Geometry: final body of the model. Coordinates: model frame, mm. Face numbers are marked on the shaded views. Give positions to 0.01 mm unless a question says otherwise; leave off trailing zeros. Loops run counter-clockwise (first coordinate to the right, second up) from the corner with the lowest first, then second, coordinate; pieces in that order, holes last. Notation, with made-up numbers: M -23,66 L 15,66 A32 cw 15,96 Z; hole C 67.25,50.25 d9. An arc over 180 degrees is marked long. Put each result on its own line as item: value.
```python
from build123d import *

# Parameters (mm, degrees)
F0_W     = 50.8
F0_H     = 101.6
F0_R     = 7.62
F1_DEPTH = 12.7
F2_R     = 5.08
F3_R     = 5.313605
F4_DEPTH = 25.4


with BuildPart() as f1:
    # F0 (on Front) → F1 (new body, symmetric)
    with BuildSketch(Plane.XZ):
        Rectangle(F0_W, F0_H)
        with Locations((0, -28.090851)):
            Circle(F0_R, mode=Mode.SUBTRACT)
        with Locations((0, 28.090851)):
            Circle(F0_R, mode=Mode.SUBTRACT)
    extrude(amount=F1_DEPTH, both=True)

    # F2
    f2_edges = [f1.edges().sort_by_distance(p)[0] for p in [
        (25.4, 0, 50.8),
        (-25.4, 0, 50.8),
        (25.4, 0, -50.8),
        (-25.4, 0, -50.8),
    ]]
    fillet(f2_edges, radius=F2_R)

    # F3 (on face) → F4 (cut, through all)
    with BuildSketch(Plane.XZ.offset(12.7)):
        with Locations((-16.311834, 41.098528)):
            Circle(F3_R)
        with Locations((16.311834, 41.098528)):
            Circle(F3_R)
        with Locations((16.311834, -41.098528)):
            Circle(F3_R)
        with Locations((-16.311834, -41.098528)):
            Circle(F3_R)
    extrude(amount=-F4_DEPTH, mode=Mode.SUBTRACT)


solid = f1.part
```
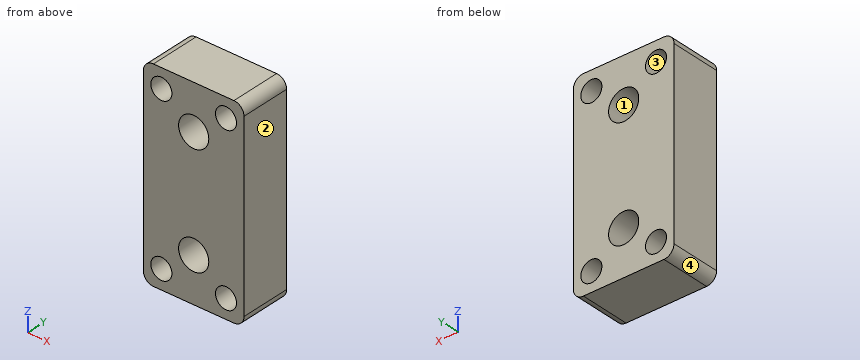
Item 1: Section C-C on z = -23. Output: boundary loops of the cut face in (x, y), then the cut area to 3 significant figures.
Output values:
outline: M -25.4,-12.7 L -5.67,-12.7 L -5.67,12.7 L -25.4,12.7 Z; M 5.67,-12.7 L 25.4,-12.7 L 25.4,12.7 L 5.67,12.7 Z
area: 1,000 mm²
Item 2: Section A-A on x = 17. Output: boundary loops of the cut face in (y, z).
Output values:
outline: M -12.7,-50.8 L 12.7,-50.8 L 12.7,-46.37 L -12.7,-46.37 Z; M -12.7,-35.83 L 12.7,-35.83 L 12.7,35.83 L -12.7,35.83 Z; M -12.7,46.37 L 12.7,46.37 L 12.7,50.8 L -12.7,50.8 Z
Item 3: Section B-B on z = 43.5. Output: boundary loops of the cut face in (x, y), then the cut area to 3 significant figures.
Output values:
outline: M -25.4,-12.7 L -21.05,-12.7 L -21.05,12.7 L -25.4,12.7 Z; M -11.57,-12.7 L 11.57,-12.7 L 11.57,12.7 L -11.57,12.7 Z; M 21.05,-12.7 L 25.4,-12.7 L 25.4,12.7 L 21.05,12.7 Z
area: 809 mm²
Item 4: Line query: probe 1 along Z at (x, y) = (0, -1.25); probe 2 along X at (y, z) = (-1, -28); probe 3 along Z at (x, y) = (1, 2). Output: solid intervals per line, ascending. Write a range as [from, to].
Output values:
probe 1: [-50.8, -35.71], [-20.47, 20.47], [35.71, 50.8]
probe 2: [-25.4, -7.62], [7.62, 25.4]
probe 3: [-50.8, -35.64], [-20.54, 20.54], [35.64, 50.8]
Item 5: Mould query, pull axis Z, two halves, no side actions, for the marked faces 1, 2, 3 and 4. Classes: pulls with the +Z half, pulls with the -Z half, needs draft (parallel to the pull), parting line crosses it, or undercut.
Output values:
face 1: undercut
face 2: needs draft
face 3: undercut
face 4: pulls with the -Z half
Item 6: Section D-D on y = 9.25. Output: boundary loops of the cut face in (x, z).
Output values:
outline: M -25.4,-45.72 A5.08 ccw -20.32,-50.8 L 20.32,-50.8 A5.08 ccw 25.4,-45.72 L 25.4,45.72 A5.08 ccw 20.32,50.8 L -20.32,50.8 A5.08 ccw -25.4,45.72 Z; hole C -16.31,-41.1 d10.63; hole C -16.31,41.1 d10.63; hole C 0,-28.09 d15.24; hole C 0,28.09 d15.24; hole C 16.31,-41.1 d10.63; hole C 16.31,41.1 d10.63
Item 7: Pin query (flat end, axial travel): pin 1 Ø13.5 at (x, z) = (0, -28.09) entering from -Y. Return the tip coordinate at first contact, or that it passes through.
Output values:
pin 1: through
